Here's how the part is built. I have some questions about the finished solid (model axes, mm). Face numbers are marked on the shaded views. A direction names the side the tool comes from. Round coordinates to 2 decimals unless told otherwise and drop trailing zeros. Write each loop counter-clockwise with the first axis right and the second up, starting at its lowest first coordinate (ties: lowest second). Pieces come first, ordered by that corner, then holes. Notation, with made-up numbers: (-26, -4) -> (16, -4) arc R5 ccw to (16, 1) -> close; hole circle Ø3 at (-17.5, 11.25). An arc over 180 degrees is marked (long way). Answer in a Markdown table with one row per item.
Autodesk Fusion 360 part; units mm, degrees
sphere "球体基本要素2" add diameter 25 placed x (0, 0, -1) y (0, 1, 0) z (1, 0, 0) at (0, 27.5, 0)
ref_plane "工作平面1" through (0, 27.5, 0) normal (0, 1, 0) x (0, 0, 1)
sketch "草图6" plane through (0, 27.5, 0) normal (0, 1, 0) x (1, 0, 0)
  circle A0 centre (8, 0) radius 1.5
  circle A1 centre (8, 0) radius 2.5
  dimension "d25" = 3
  dimension "d26" = 5
  dimension "d27" = 8
extrude "拉伸6" cut sketch "草图6" along normal through all
extrude "拉伸7" cut sketch "草图6" along normal blind 16 contours A0
extrude "拉伸8" add sketch "草图6" along normal blind 8 contours A0
thread "螺纹3"
sketch "草图7" plane through (0, 0, 0) normal (0, 0, 1) x (1, 0, 0)
  line L0 (-0.0753, 40.4285) -> (-0.0753, 14.5)
  line L1 (-0.0753, 14.5) -> (-0.0753, 40.5)
  line L2 (-0.0753, 40.5) -> (-0.0753, 14.5)
  dimension "d33" = 26
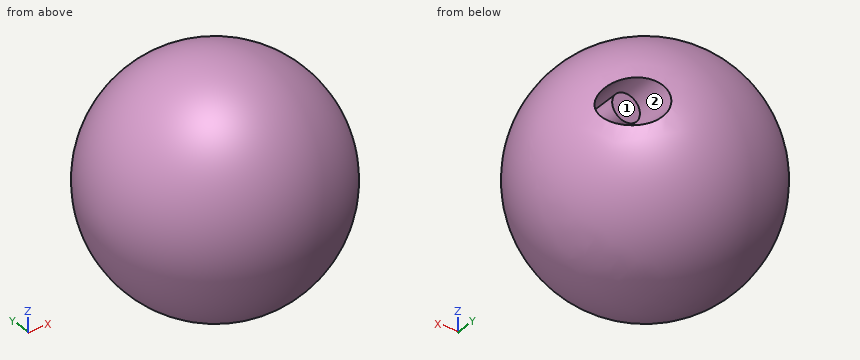
1) I want a section at C-C, the plane z = 0. List the corners of the cut face in (x, y) for me, and give its area (3 significant figures).
Response:
| item | result |
|---|---|
| outline | (5.5, 27.5) -> (5.5, 38.72) arc R12.5 ccw (long way) to (10.5, 34.28) -> (10.5, 27.5) -> (9.5, 27.5) -> (9.5, 35.5) -> (6.5, 35.5) -> (6.5, 27.5) -> close |
| area | 468 mm^2 |
2) Which directions (+Z, -Z, +X, -X, +Y, -Y) give clear straight access to the entire face, cutting with the end or side of a thin tool? Please do the marked faces 1 and 2.
Response:
| item | result |
|---|---|
| face 1 | +X, +Y |
| face 2 | +Y |
3) For pin 1 (1 mm diameter, centred on x = 1, y = 25, fed in from +Z); pin 2 (2 mm diameter, centred on x = 0.5, y = 25, fed in from +Z); pin 3 (8 mm diameter, centred on y = 21.5, z = -1, fed in from -X), each with a flat end and sliding along its axis, tell me the tip position at first contact or that it passes through.
Response:
| item | result |
|---|---|
| pin 1 | stops at z = 12.31 |
| pin 2 | stops at z = 12.4 |
| pin 3 | stops at x = -12.33 |
4) I want a section at D-D, the plane y = 24. List the corners of the cut face in (x, z) for me, and give its area (3 significant figures).
Response:
| item | result |
|---|---|
| outline | circle Ø24 at (0, 0) |
| area | 452 mm^2 |
5) I want a section at A-A, the plane y = 29.5. List the corners of the cut face in (x, z) for me, and give its area (3 significant figures).
Response:
| item | result |
|---|---|
| outline | circle Ø24.68 at (0, 0); circle Ø3 at (8, 0); hole circle Ø5 at (8, 0) |
| area | 466 mm^2 |
6) I need wall thicknesses on line 1 (X direction, y = 30, z = 0); line 2 (X direction, y = 30.5, z = 0); line 3 (Z direction, x = 8, y = 31). Which ranges of each line are inside material? Lowest first, please. Write a range as [from, to].
Response:
| item | result |
|---|---|
| line 1 | x = [-12.25, 5.5], [6.5, 9.5], [10.5, 12.25] |
| line 2 | x = [-12.13, 5.5], [6.5, 9.5], [10.5, 12.13] |
| line 3 | z = [-8.94, -2.5], [-1.5, 1.5], [2.5, 8.94] |
7) I want a section at B-B, the plane x = 8.25. List the corners of the cut face in (y, z) for me.
Response:
| item | result |
|---|---|
| outline | (27.5, -2.49) -> (27.5, -1.48) -> (35.5, -1.48) -> (35.5, 1.48) -> (27.5, 1.48) -> (27.5, 2.49) -> (36.56, 2.49) arc R9.39 ccw (long way) to (36.56, -2.49) -> close |
